```python
from build123d import *

# Parameters (mm, degrees)
SKETCH3_R                = 3
CUT_EXTRUDE1_DEPTH       = 18.5
SKETCH5_R                = 1.5
CUT_EXTRUDE3_DEPTH       = 10
CIRPATTERN1_COUNT        = 2
CIRPATTERN1_ANGLE        = 90
CUT_EXTRUDE2_DEPTH       = 10
FILLET1_R                = 0.6
CIRPATTERN2_COUNT        = 12
FILLET1_OF_CIRPATTERN2_R = 0.6


with BuildPart() as part:
    # Sketch2 → Revolve1 (revolve)
    with BuildSketch(Plane.XY):
        Polygon((0, 0), (0, 7.5), (0.5, 7.5), (0.5, 5.73), (10.5, 5.73), (10.5, 7.5), (17.5, 7.5), (17.5, 0), align=None)
    revolve(axis=Axis((19.21222629, 0, 0), (-1, 0, 0)))

    # Sketch3 → Cut-Extrude1 (cut, through all)
    with BuildSketch(Plane.ZY):
        Circle(SKETCH3_R)
    extrude(amount=-CUT_EXTRUDE1_DEPTH, mode=Mode.SUBTRACT)

    # Sketch5 → Cut-Extrude3 (cut)
    with BuildSketch(Plane(origin=(0, 0, 0), x_dir=(1, 0, 0), z_dir=(0, 1, 0))):
        with Locations((14, 0)):
            Circle(SKETCH5_R)
    cut_extrude3 = extrude(amount=CUT_EXTRUDE3_DEPTH, mode=Mode.SUBTRACT)

    # CirPattern1: Cut-Extrude3 ×2 about axis
    cirpattern1_axis = Axis((19.21222629, 0, 0), (1, 0, 0))
    for i in range(1, CIRPATTERN1_COUNT):
        add(cut_extrude3.rotate(cirpattern1_axis, i * CIRPATTERN1_ANGLE / (CIRPATTERN1_COUNT - 1)), mode=Mode.SUBTRACT)

    # Sketch4 → Cut-Extrude2 (cut)
    with BuildSketch(Plane(origin=(0.5, 0, 0), x_dir=(0, 0, -1), z_dir=(1, 0, 0))):
        Polygon((1.125, 7.23), (-1.125, 7.23), (-0.5625, 4.23), (0.5625, 4.23), align=None)
    cut_extrude2 = extrude(amount=CUT_EXTRUDE2_DEPTH, mode=Mode.SUBTRACT)

    # Fillet1
    fillet1_edges = [part.edges().sort_by_distance(p)[0] for p in [
        (5.5, 5.669222732, -0.832354262),
        (5.5, 4.23, -0.5625),
        (5.5, 5.669222732, 0.832354262),
        (5.5, 4.23, 0.5625),
    ]]
    fillet(fillet1_edges, radius=FILLET1_R)

    # CirPattern2: Cut-Extrude2 ×12 about axis
    cirpattern2_axis = Axis((0, 0, 0), (1, 0, 0))
    for i in range(1, CIRPATTERN2_COUNT):
        add(cut_extrude2.rotate(cirpattern2_axis, i * 360 / CIRPATTERN2_COUNT), mode=Mode.SUBTRACT)

    # Fillet1 of CirPattern2
    fillet1_of_cirpattern2_edges = [part.edges().sort_by_distance(p)[0] for p in [
        (5.5, 5.325868037, 2.11377143),
        (5.5, 3.944537458, 1.62786071),
        (5.5, 4.493513774, 3.555451302),
        (5.5, 3.382037458, 2.60213929),
        (5.5, 3.555451302, 4.493513774),
        (5.5, 2.60213929, 3.382037458),
        (5.5, 2.11377143, 5.325868037),
        (5.5, 1.62786071, 3.944537458),
        (5.5, 0.832354262, 5.669222732),
        (5.5, 0.5625, 4.23),
        (5.5, -0.832354262, 5.669222732),
        (5.5, -0.5625, 4.23),
        (5.5, -2.11377143, 5.325868037),
        (5.5, -1.62786071, 3.944537458),
        (5.5, -3.555451302, 4.493513774),
        (5.5, -2.60213929, 3.382037458),
        (5.5, -4.493513774, 3.555451302),
        (5.5, -3.382037458, 2.60213929),
        (5.5, -5.325868037, 2.11377143),
        (5.5, -3.944537458, 1.62786071),
        (5.5, -5.669222732, 0.832354262),
        (5.5, -4.23, 0.5625),
        (5.5, -5.669222732, -0.832354262),
        (5.5, -4.23, -0.5625),
        (5.5, -5.325868037, -2.11377143),
        (5.5, -3.944537458, -1.62786071),
        (5.5, -4.493513774, -3.555451302),
        (5.5, -3.382037458, -2.60213929),
        (5.5, -3.555451302, -4.493513774),
        (5.5, -2.60213929, -3.382037458),
        (5.5, -2.11377143, -5.325868037),
        (5.5, -1.62786071, -3.944537458),
        (5.5, -0.832354262, -5.669222732),
        (5.5, -0.5625, -4.23),
        (5.5, 0.832354262, -5.669222732),
        (5.5, 0.5625, -4.23),
        (5.5, 2.11377143, -5.325868037),
        (5.5, 1.62786071, -3.944537458),
        (5.5, 3.555451302, -4.493513774),
        (5.5, 2.60213929, -3.382037458),
        (5.5, 4.493513774, -3.555451302),
        (5.5, 3.382037458, -2.60213929),
        (5.5, 5.325868037, -2.11377143),
        (5.5, 3.944537458, -1.62786071),
    ]]
    fillet(fillet1_of_cirpattern2_edges, radius=FILLET1_OF_CIRPATTERN2_R)


solid = part.part
```
Model file for the job. Use its own axes, mm. A direction names the side the tool comes from. Coordinates: 2 decimals unless noted, no trailing zeros. Loops run counter-clockwise (first coordinate to the right, second up) from the corner with the lowest first, then second, coordinate; pieces in that order, holes last. Notation, with made-up numbers: (32, 46) - (39, 46) arc R24 cw to (39, 79) - close; hole circle Ø5 at (29, 74.5). An arc over 180 degrees is marked (long way). Answer as a JSON object with one key per item and string values. Group by question number.
(1) Tool access for faces 4 (the face through (5.57, -4.24, -3.6)), 5 (the face through (10.5, 0, 5)), 6 (the face through (13.805, 5.015, -1.487)): list every direction of +Z, -Z, +X, -X, +Y, -Y with a clear straight run to the whole face (end or side of a thin tool).
(2) Cut at C-C (y = -6.5). Give the cut face in (x, z), then the cut area to 3 significant figures.
(3) Flat gauge pins, fed straight in: pin 1 (1 mm diameter, centred on x = 4.5, y = -2.5, fed in from -Z); pin 2 (2.5 mm diameter, centred on x = 14, y = 0, fed in from +Z); pin 3 (3 mm diameter, centred on x = 2.5, z = 0.5, fed in from +Y); pin 4 (3.5 mm diameter, centred on y = 0, z = 0, fed in from -X). Where does each tip first touch, or does it go through?
(4) Cut at A-A (y = -2.5). Give the cut face in (x, z).
(5) Probe line 1 along X through (y, z) = (4.5, 3.5); line 2 along X through (y, z) = (4.4, 0); line 3 along Y through (x, z) = (6.75, -4.5). List the from-to ranges inside material, lowest first.
(6) Two-plate mould, pull along Y, no slides. Class faces 1 (the face through (5.57, 3.6, -4.24)), 2 (the face through (5.57, 4.24, 3.6)), 3 (the face through (14.049, -7.493, -0.33)): released by +Y, released by -Y, zero draft, split by the parting line, or undercut.
(7) Cut at B-B (x = 14.5). Give the cut face in (y, z), then the cut area to 3 significant figures.
Geometry says:
{
 "1": {"face 4": "-Y", "face 5": "none", "face 6": "+Y"},
 "2": {"outline": "(0, -3.74) - (0.5, -3.74) - (0.5, 3.74) - (0, 3.74) - close; (10.5, -3.74) - (17.5, -3.74) - (17.5, 3.74) - (10.5, 3.74) - close", "area": "56.1 mm^2"},
 "3": {"pin 1": "stops at z = -3.85", "pin 2": "stops at z = -2.73", "pin 3": "stops at y = 5.56", "pin 4": "passes through"},
 "4": {"outline": "(0, -7.07) - (0.5, -7.07) - (0.5, -3.55) - (10.5, -3.55) - (10.5, -7.07) - (17.5, -7.07) - (17.5, -1.66) - (0, -1.66) - close; (0, 1.66) - (17.5, 1.66) - (17.5, 7.07) - (10.5, 7.07) - (10.5, 3.55) - (0.5, 3.55) - (0.5, 7.07) - (0, 7.07) - close"},
 "5": {"line 1": "x = 0 to 0.5, 10.5 to 17.5", "line 2": "x = 0 to 0.5, 10.5 to 12.5, 15.5 to 17.5", "line 3": "y = -1.82 to -0.57, 0.57 to 1.82"},
 "6": {"face 1": "undercut", "face 2": "released by +Y", "face 3": "split by the parting line"},
 "7": {"outline": "(-1.41, 2.65) - (-1.41, 7.37) arc R7.5 ccw (long way) to (7.37, -1.41) - (2.65, -1.41) arc R3 cw (long way) to start; (1.41, 2.65) arc R3 cw to (2.65, 1.41) - (7.37, 1.41) arc R7.5 ccw to (1.41, 7.37) - close", "area": "123 mm^2"}
}
